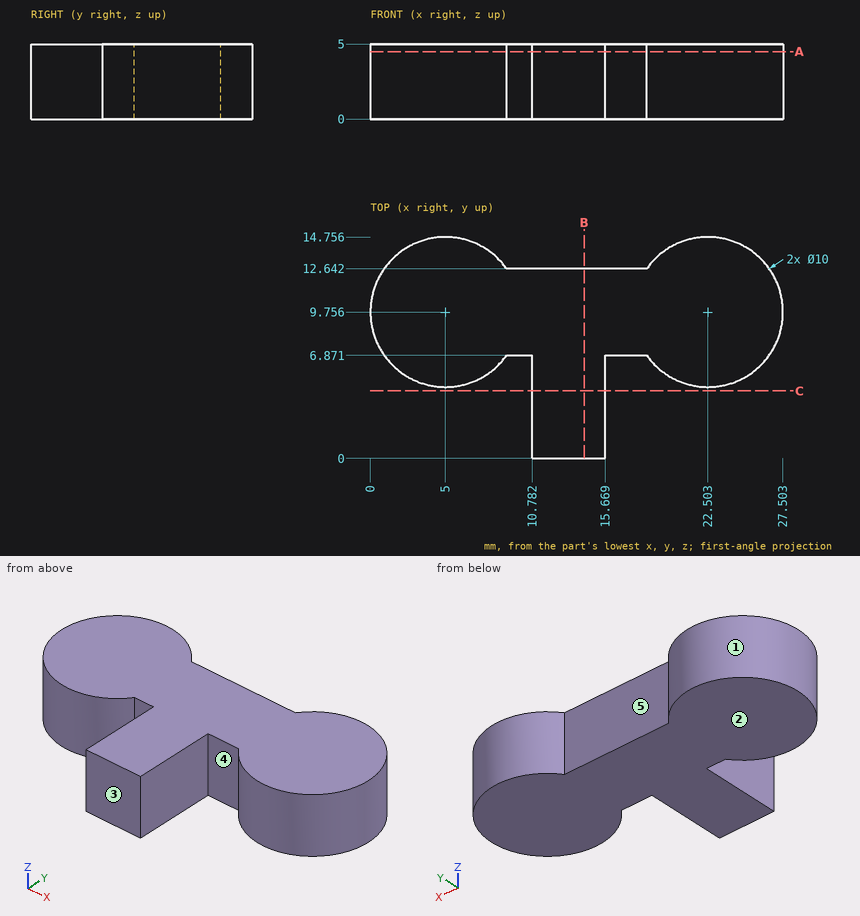
The figure shows three views and two pictorial views of one solid part (mm, origin at its lowest corner). Answer the questions. A direction names the side the tool comes from. Coordinates: 2 decimals unless noted, no trailing zeros. Loops run counter-clockwise (first coordinate to the right, second up) from the corner with the lowest first, then second, coordinate; pieces in that order, holes last.
(1) The part is cut by section C-C (y = 4.5). Determine the outline of the cut face in (x, z).
Solution:
outline: (10.78, 0) - (15.67, 0) - (15.67, 5) - (10.78, 5) - close
(2) The mould has two halves that part along X. Classify the marked faces 1 and 2: released by +X, released by -X, zero draft, split by the parting line, or undercut.
Solution:
face 1: undercut
face 2: zero draft
(3) A tool of negligible diameter and unlimited length cuts with its end or side. For the marked faces 3, 4 and 5, from which of +Z, -Z, +X, -X, +Y, -Y can it reach the whole face along a straight path? Write none if from no direction.
Solution:
face 3: +Z, -Z, +X, -X, -Y
face 4: +Z, -Z, -Y
face 5: +Z, -Z, +Y
(4) Consider line 1 along X through (y, z) = (6.75, 3.7) (1 decimal); line 2 along X through (y, z) = (1.75, 3.9); line 3 along X through (y, z) = (14.25, 1.9) (1 decimal). Determine where each line is inside the solid, lowest interval first.
Solution:
line 1: x = 1 to 9, 10.8 to 15.7, 18.5 to 26.5
line 2: x = 10.78 to 15.67
line 3: x = 2.8 to 7.2, 20.3 to 24.7
(5) The part is cut by section B-B (x = 14.25). Determine the outline of the cut face in (y, z).
Solution:
outline: (0, 0) - (12.64, 0) - (12.64, 5) - (0, 5) - close
(6) Flat-ended cylindrical pins translate along their axes: pin 1 Ø3 at (x, z) = (19, 2.5) entering from -Y (1 decimal); pin 2 Ø2.5 at (y, z) = (2.5, 2.5) entering from -X; pin 3 Ø1.5 at (x, z) = (16, 3) entering from +Y. Find the tip coordinate at first contact, or state that the pin passes through.
Solution:
pin 1: stops at y = 5.2
pin 2: stops at x = 10.78
pin 3: stops at y = 12.64
(7) The part is cut by section A-A (z = 4.5). Determine the outline of the cut face in (x, y), and give its area (3 significant figures).
Solution:
outline: (9.08, 6.87) - (10.78, 6.87) - (10.78, 0) - (15.67, 0) - (15.67, 6.87) - (18.42, 6.87) arc R5 ccw (long way) to (18.42, 12.64) - (9.08, 12.64) arc R5 ccw (long way) to start
area: 237 mm2
